from build123d import *

# Parameters (mm, degrees)
F1_DEPTH = 600
F2_T     = -2.54
F3_W     = 50
F3_H     = 50
F5_W     = 50
F5_H     = 50


with BuildPart() as f1:
    # F0 (on Front) → F1 (new body)
    with BuildSketch(Plane.XZ):
        Polygon((300, 25.4), (-300, 25.4), (-300, 0), (-250, 0), (250, 0), (300, 0), align=None)
    extrude(amount=F1_DEPTH)

    # F2
    f2_openings = [f1.faces().sort_by_distance(p)[0] for p in [
        (0, -300, 25.4),
    ]]
    offset(amount=F2_T, openings=f2_openings)

    # F3 (on face) → F6 section 0
    with BuildSketch(Plane(origin=(0, 0, 0), x_dir=(1, 0, 0), z_dir=(0, 0, -1))):
        with Locations((-225, 525)):
            Rectangle(F3_W, F3_H)
    # F5 (on offset) → F6 section 1
    with BuildSketch(Plane.XY.offset(-800)):
        with Locations((-277.383376, -523.17366)):
            Rectangle(F5_W, F5_H)
    loft()


solid = f1.part
Model file for the job. Use its own axes, mm. A direction names the side the tool comes from. Round coordinates to 2 decimals unless told otherwise and drop trailing zeros. Order: outer loops, then holes, each group sorted by start corner. A loop starts at its lowest first (then second) coordinate and runs counter-clockwise, first axis right, second up.
(1) Band-saw the part on B-B (y = -77.5). List the corners of the cut face in (x, z).
(2) Drill centre lines: line 1 (Z direction, x = -61, y = -52.5); line 2 (Y direction, x = -254.5, z = -279.5); line 3 (Y direction, x = -250, z = -496.5). Where is each one in solid material? Low to high.
(3) Band-saw the part on A-A (x = -21.5). List the corners of the cut face in (y, z), then the cut area to 3 significant figures.
(4) Pin check, flat tips, straight feed: pin 1 (25 mm diameter, centred on y = -334.5, z = 16.5, fed in from -X); pin 2 (7 mm diameter, centred on x = 48.5, z = 19.5, fed in from +Y); pin 3 (5 mm diameter, centred on x = 149, y = -454, fed in from -Z). Stop position of each tip, or through.
(5) 3-axis set-ups, long thin cutter, end or side, ignore diameter. For faces 1 (the face through (-4, -2.54, 14)), 2 (the face through (-278, -523, -800)): which of +Z, -Z, +X, -X, +Y, -Y reach the whole face in a straight line?
(6) Pull direction X, two halves, no side cores. Call faces 3 (the face through (-4, -597.46, 14)), 4 (the face through (300, -296, 13)), 5 (the face through (-4, 0, 13)): released by +X, released by -X, zero draft, split by the parting line, or undercut.
Verdict:
1. outline: (-300, 0) - (300, 0) - (300, 25.4) - (297.46, 25.4) - (297.46, 2.54) - (-297.46, 2.54) - (-297.46, 25.4) - (-300, 25.4) - close
2. line 1: z = 0 to 2.54
2. line 2: y = -549.36 to -499.36
2. line 3: y = -548.87 to -498.87
3. outline: (-600, 0) - (0, 0) - (0, 25.4) - (-2.54, 25.4) - (-2.54, 2.54) - (-597.46, 2.54) - (-597.46, 25.4) - (-600, 25.4) - close
3. area: 1,640 mm2
4. pin 1: stops at x = -300
4. pin 2: stops at y = 0
4. pin 3: stops at z = 0
5. face 1: +Z
5. face 2: -Z, +X, -X, +Y, -Y
6. face 3: undercut
6. face 4: released by +X
6. face 5: zero draft
